Verification items for the finished model (mm, model axes). A direction names the side the tool comes from. Give positions to 0.01 mm unless a question says otherwise; leave off trailing zeros. Write each loop counter-clockwise with the first axis right and the second up, starting at its lowest first coordinate (ties: lowest second). Pieces come first, ordered by that corner, then holes. Notation, with made-up numbers: (37, -38) - (59, -38) arc R33 cw to (59, -3) - close; hole circle Ø10 at (6.5, 69.5). An arc over 180 degrees is marked (long way). Answer as a JSON object with one key per item and string values. Group by question number.
Item 1: Sectioned sample at A-A, the plane y = -3.55. Count the separate pieces of the cut face and the enclosed holes in it, and give its area (3 significant figures).
Item 2: Sectioned sample at D-D, the plane z = -19. Record the boundary of the cut face in (x, y).
Item 3: Scan lines: line 1 along X through (y, z) = (-3.85, 82.5); line 2 along Z through (x, y) = (6.5, -1.85); line 3 along X through (y, z) = (-1.25, 68.5). Record each from-to range of solid material in increasing order. Write a range as [from, to].
Item 4: Tool access check on faces 4 (the face through (0, -5, -38)), 5 (the face through (4, -2, -9)), 6 (the face through (-8, -2, -110)). Record the directions out of +Z, -Z, +X, -X, +Y, -Y that give a thin tool (end or side, any length) a straight path to the whole face; none if there is none.
Item 5: Sectioned sample at C-C, the plane x = 8.5. Record the boundary of the cut face in (y, z).
Item 6: Sectioned sample at B-B, the plane z = -113. Record the boundary of the cut face in (x, y).
Item 7: Go/stop test with flat-tipped pins: pin 1 (2.5 mm diameter, centred on x = 0, z = 82.5, fed in from -Y); pin 2 (1.5 mm diameter, centred on x = 7, y = -2.5, fed in from +Z); pin 3 (2 mm diameter, centred on y = -3.5, z = -9, fed in from +X). Record where each tip stops, or that it passes through.
Item 8: Draft check along Z on faces 1 (the face through (1.075, -2.465, -111.314)), 2 (the face through (0, -2, -125)), 3 (the face through (-12, -2, -117)). Enter one of: +Z half, -Z half, draft (parallel to the pull), parting line (faces both ways), or undercut.
```python
from build123d import *

# Parameters (mm, degrees)
F0_R     = 2
F0_R_2   = 1.3
F1_DEPTH = 5


with BuildPart() as f1:
    # F0 (on Front) → F1 (new body)
    with BuildSketch(Plane.XZ):
        Polygon((-4, -125), (4, -125), (12, -125), (12, -110), (4, -110), (4, 95), (-4, 95), (-4, -110), (-12, -110), (-12, -125), align=None)
        with Locations((0, -121)):
            Circle(F0_R, mode=Mode.SUBTRACT)
        with Locations((0, -113)):
            Circle(F0_R, mode=Mode.SUBTRACT)
        with Locations((0, 27.5)):
            Circle(F0_R_2, mode=Mode.SUBTRACT)
        with Locations((0, 32.5)):
            Circle(F0_R_2, mode=Mode.SUBTRACT)
        with Locations((0, 37.5)):
            Circle(F0_R_2, mode=Mode.SUBTRACT)
        with Locations((0, 42.5)):
            Circle(F0_R_2, mode=Mode.SUBTRACT)
        with Locations((0, 47.5)):
            Circle(F0_R_2, mode=Mode.SUBTRACT)
        with Locations((0, 52.5)):
            Circle(F0_R_2, mode=Mode.SUBTRACT)
        with Locations((0, 57.5)):
            Circle(F0_R_2, mode=Mode.SUBTRACT)
        with Locations((0, 62.5)):
            Circle(F0_R_2, mode=Mode.SUBTRACT)
        with Locations((0, 67.5)):
            Circle(F0_R_2, mode=Mode.SUBTRACT)
        with Locations((0, 72.5)):
            Circle(F0_R_2, mode=Mode.SUBTRACT)
        with Locations((0, 77.5)):
            Circle(F0_R_2, mode=Mode.SUBTRACT)
        with Locations((0, 82.5)):
            Circle(F0_R_2, mode=Mode.SUBTRACT)
        with Locations((0, 87.5)):
            Circle(F0_R_2, mode=Mode.SUBTRACT)
        with Locations((0, 92.5)):
            Circle(F0_R_2, mode=Mode.SUBTRACT)
    extrude(amount=F1_DEPTH)


solid = f1.part
```
Geometry check:
{
 "1": {"separate pieces": "1", "enclosed holes": "16", "area": "1,900 mm^2"},
 "2": {"outline": "(-4, -5) - (4, -5) - (4, 0) - (-4, 0) - close"},
 "3": {"line 1": "[-4, -1.3], [1.3, 4]", "line 2": "[-125, -110]", "line 3": "[-4, -0.83], [0.83, 4]"},
 "4": {"face 4": "+Z, -Z, +X, -X, -Y", "face 5": "+Z, +X, +Y, -Y", "face 6": "+Z, -X, +Y, -Y"},
 "5": {"outline": "(-5, -125) - (0, -125) - (0, -110) - (-5, -110) - close"},
 "6": {"outline": "(-12, -5) - (-2, -5) - (-2, 0) - (-12, 0) - close; (2, -5) - (12, -5) - (12, 0) - (2, 0) - close"},
 "7": {"pin 1": "through", "pin 2": "z = -110", "pin 3": "x = 4"},
 "8": {"face 1": "undercut", "face 2": "-Z half", "face 3": "draft"}
}
